```python
from build123d import *

# Parameters (mm, degrees)
F0_R     = 2
F0_R_2   = 40
F1_DEPTH = 3
F0_W     = 8
F0_H     = 9
F0_R_3   = 1.5
F0_W_2   = 6
F0_W_3   = 9
F2_DEPTH = 26
F3_R     = 2


with BuildPart() as f1:
    # F0 (on Front) → F1 (new body)
    with BuildSketch(Plane.XZ):
        Polygon((41, -46), (46, -46), (46, 46), (41, 46), (-41, 46), (-46, 46), (-46, -46), (-41, -46), align=None)
        with Locations((-41, -41)):
            Circle(F0_R, mode=Mode.SUBTRACT)
        with Locations((41, -41)):
            Circle(F0_R, mode=Mode.SUBTRACT)
        with Locations((-41, 41)):
            Circle(F0_R, mode=Mode.SUBTRACT)
        Circle(F0_R_2, mode=Mode.SUBTRACT)
        with Locations((41, 41)):
            Circle(F0_R, mode=Mode.SUBTRACT)
        Polygon((41, -54), (41, -46), (-41, -46), (-41, -54), (-32, -54), (-32, -63), (32, -63), (32, -54), align=None)
        Polygon((-41, 46), (41, 46), (41, 54), (35, 54), (35, 63), (-33, 63), (-33, 54), (-41, 54), align=None)
    extrude(amount=F1_DEPTH)

    # F0 (on Front) → F2 (join)
    with BuildSketch(Plane.XZ):
        with Locations((-37, 58.5)):
            Rectangle(F0_W, F0_H)
        with Locations((-37, 59)):
            Circle(F0_R_3, mode=Mode.SUBTRACT)
        with Locations((38, 58.5)):
            Rectangle(F0_W_2, F0_H)
        with Locations((37, 59)):
            Circle(F0_R_3, mode=Mode.SUBTRACT)
        with Locations((36.5, -58.5)):
            Rectangle(F0_W_3, F0_H)
        with Locations((37, -59)):
            Circle(F0_R_3, mode=Mode.SUBTRACT)
        with Locations((-36.5, -58.5)):
            Rectangle(F0_W_3, F0_H)
        with Locations((-37, -59)):
            Circle(F0_R_3, mode=Mode.SUBTRACT)
    extrude(amount=F2_DEPTH)

    # F3
    f3_edges = [f1.edges().sort_by_distance(p)[0] for p in [
        (-40, -3, 0),
        (-46, -1.5, -46),
        (-46, -1.5, 46),
        (46, -1.5, -46),
        (41, -1.5, -46),
        (-41, -1.5, -46),
        (-41, -13, -63),
        (41, -13, -63),
        (46, -1.5, 46),
        (41, -1.5, 46),
        (41, -13, 63),
        (-41, -13, 63),
        (-41, -1.5, 46),
    ]]
    fillet(f3_edges, radius=F3_R)


solid = f1.part
```
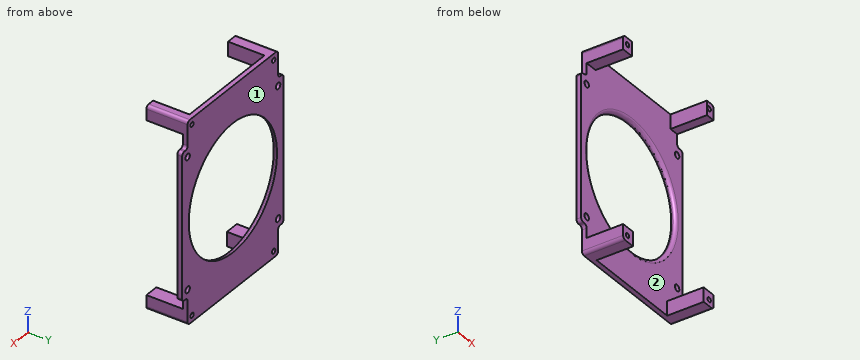
CAD build for the part. Positions are in the model's coordinates, mm. Face numbers are marked on the shaded views. Round coordinates to 2 decimals unless told otherwise and drop trailing zeros. Write each loop counter-clockwise with the first axis right and the second up, starting at its lowest first coordinate (ties: lowest second). Pieces come first, ordered by that corner, then holes. Notation, with made-up numbers: (-25, 31.5) - (14, 31.5) arc R22 cw to (14, 40.5) - close; hole circle Ø1 at (-28, 89.5). An arc over 180 degrees is marked (long way). Return JSON: item names as keys, results as strings. Group by question number.
Item 1: Band-saw the part on B-B on z = 59. List the corners of the cut face in (x, y), plus the area to 3 significant figures.
Item 2: Flat gauge pins, fed straight in: pin 1 Ø12 at (x, z) = (-34, 26) entering from +Y; pin 2 Ø0.5 at (x, y) = (43.5, -1.5) entering from +Z; pin 3 Ø10.5 at (y, z) = (-9, -52) entering from +X; pin 4 Ø10.5 at (y, z) = (-8.5, 56.5) entering from -X. Where does each tip first touch, or does it go through?
Item 3: Band-saw the part on A-A on y = -15. List the corners of the cut face in (x, z).
Item 4: Probe probe 1 along Z at (x, y) = (37, -16.75); probe 2 along Z at (x, y) = (-39, -13); probe 3 along Z at (x, y) = (0, -0.55). List the from-to ranges inside material, lowest first.
Item 5: Band-saw the part on C-C on x = 37. State how many separate pieces and enclosed holes the cut face has, plus the area to 3 significant figures.
Item 6: Mould opens along X. For the marked faces 1 and 2 say: +X half, -X half, draft (parallel to the pull), parting line (faces both ways), or undercut.
Resolved:
{
 "1": {"outline": "(-41, -26) - (-38.5, -26) - (-38.5, 0) - (-41, 0) - close; (-35.5, -26) - (-33, -26) - (-33, -3) - (35, -3) - (35, -26) - (35.5, -26) - (35.5, 0) - (-35.5, 0) - close; (38.5, -26) - (41, -26) - (41, 0) - (38.5, 0) - close", "area": "412 mm²"},
 "2": {"pin 1": "stops at y = 0", "pin 2": "stops at z = 46", "pin 3": "stops at x = 41", "pin 4": "stops at x = -41"},
 "3": {"outline": "(-41, -61) arc R2 ccw to (-39, -63) - (-32, -63) - (-32, -54) - (-41, -54) - close; (-41, 54) - (-33, 54) - (-33, 63) - (-39, 63) arc R2 ccw to (-41, 61) - close; (32, -63) - (39, -63) arc R2 ccw to (41, -61) - (41, -54) - (32, -54) - close; (35, 54) - (41, 54) - (41, 61) arc R2 ccw to (39, 63) - (35, 63) - close; hole circle Ø3 at (-37, -59); hole circle Ø3 at (-37, 59); hole circle Ø3 at (37, -59); hole circle Ø3 at (37, 59)"},
 "4": {"probe 1": "z = -63 to -60.5, -57.5 to -54, 54 to 57.5, 60.5 to 63", "probe 2": "z = -63 to -54, 54 to 63", "probe 3": "z = -63 to -40, 40 to 63"},
 "5": {"separate pieces": "4", "enclosed holes": "0", "area": "541 mm²"},
 "6": {"face 1": "draft", "face 2": "undercut"}
}
